```python
from build123d import *

# Parameters (mm, degrees)
BOSS_EXTRUDE1_DEPTH     = 22
SKETCH2_W               = 18.000000089
SKETCH2_H               = 20
BOSS_EXTRUDE2_DEPTH     = 7
SKETCH3_W               = 70
SKETCH3_H               = 50
BOSS_EXTRUDE3_DEPTH     = 4
SKETCH31_W              = 18.000000089
SKETCH31_H              = 3
BOSS_EXTRUDE7_DEPTH     = 34
CUT_EXTRUDE1_REACH      = 52
CUT_EXTRUDE_THIN1_REACH = 72
SKETCH7_W               = 25.000000089
SKETCH7_H               = 30
SKETCH8_W               = 18.000000089
SKETCH8_H               = 23
CUT_EXTRUDE2_DEPTH      = 27.000000055
CUT_EXTRUDE2_DEPTH_BACK = 45.000000145
SKETCH10_R              = 1
CUT_EXTRUDE3_DEPTH      = 10
SKETCH12_W              = 4
SKETCH12_H              = 5
CUT_EXTRUDE4_DEPTH      = 4
SKETCH13_W              = 18.000000089
SKETCH13_H              = 23
BOSS_EXTRUDE4_DEPTH     = 5
SKETCH14_R              = 1
CUT_EXTRUDE5_DEPTH      = 10
CUT_EXTRUDE6_REACH      = 40
CUT_EXTRUDE10_START     = -17
SKETCH29_W              = 13
SKETCH29_H              = 23
CUT_EXTRUDE10_DEPTH     = 17
SKETCH30_W              = 4
SKETCH30_H              = 1
CUT_EXTRUDE11_DEPTH     = 7
SKETCH21_R              = 5
CUT_EXTRUDE12_DEPTH     = 6
SKETCH32_R              = 4.999999958
BOSS_EXTRUDE8_DEPTH     = 2
CUT_EXTRUDE13_REACH     = 44.05
SKETCH33_R              = 1.5
SKETCH34_R              = 2.5
CUT_EXTRUDE14_DEPTH     = 1


with BuildPart() as part:
    # Sketch1 → Boss-Extrude1 (new body)
    with BuildSketch(Plane.XZ.offset(109.542579658)):
        Polygon((23.483775445, -24.37606884), (23.483775445, -44.37606884), (5.483775356, -44.37606884), (5.483775356, -24.37606884), (8.483775356, -24.37606884), (8.483775445, -41.37606884), (20.483775445, -41.37606884), (20.483775445, -24.37606884), align=None)
    extrude(amount=-BOSS_EXTRUDE1_DEPTH)

    # Sketch2 → Boss-Extrude2 (add)
    with BuildSketch(Plane.XZ.offset(109.542579658)):
        with Locations((14.483775401, -34.37606884)):
            Rectangle(SKETCH2_W, SKETCH2_H)
    extrude(amount=BOSS_EXTRUDE2_DEPTH)

    # Sketch3 → Boss-Extrude3 (add)
    with BuildSketch(Plane.XZ.offset(116.542579658)):
        with Locations((14.4837754, -26.325627156)):
            Rectangle(SKETCH3_W, SKETCH3_H)
    extrude(amount=BOSS_EXTRUDE3_DEPTH)

    # Sketch31 → Boss-Extrude7 (add)
    with BuildSketch(Plane(origin=(0, -116.542579658, 0), x_dir=(1, 0, 0), z_dir=(0, 1, 0))):
        with Locations((14.483775401, 45.87606884)):
            Rectangle(SKETCH31_W, SKETCH31_H)
    extrude(amount=BOSS_EXTRUDE7_DEPTH)

    # Sketch4 → Cut-Extrude1 (cut, up to next)
    with BuildSketch(Plane(origin=(0, 0, -51.325627156), x_dir=(-1, 0, 0), z_dir=(0, 0, -1)), mode=Mode.PRIVATE) as cut_extrude1_sk1:
        with BuildLine():
            Line((-49.4837754, -117.542579658), (-49.4837754, -120.542579658))
            Line((-49.4837754, -120.542579658), (-46.4837754, -120.542579658))
            ThreePointArc((-46.4837754, -120.542579658), (-48.605095744, -119.663900001), (-49.4837754, -117.542579658))
        make_face()
    cut_extrude1_tool1 = extrude(cut_extrude1_sk1.sketch, amount=-CUT_EXTRUDE1_REACH, mode=Mode.PRIVATE) & part.part
    add(cut_extrude1_tool1.solids().sort_by_distance((48.813672, -119.872476, -51.325627))[0], mode=Mode.SUBTRACT)
    # Sketch4 → Cut-Extrude1 (cut, up to next)
    with BuildSketch(Plane(origin=(0, 0, -51.325627156), x_dir=(-1, 0, 0), z_dir=(0, 0, -1)), mode=Mode.PRIVATE) as cut_extrude1_sk2:
        with BuildLine():
            Line((17.5162246, -120.542579658), (20.5162246, -120.542579658))
            Line((20.5162246, -120.542579658), (20.5162246, -117.542579658))
            ThreePointArc((20.5162246, -117.542579658), (19.637544943, -119.663900001), (17.5162246, -120.542579658))
        make_face()
    cut_extrude1_tool2 = extrude(cut_extrude1_sk2.sketch, amount=-CUT_EXTRUDE1_REACH, mode=Mode.PRIVATE) & part.part
    add(cut_extrude1_tool2.solids().sort_by_distance((-19.846121, -119.872476, -51.325627))[0], mode=Mode.SUBTRACT)

    # Sketch6 → Cut-Extrude-Thin1 (cut, up to next)
    with BuildSketch(Plane.ZY.offset(20.5162246), mode=Mode.PRIVATE) as cut_extrude_thin1_sk1:
        with BuildLine():
            ThreePointArc((-4.325627156, -120.542579658), (-2.204306812, -119.663900001), (-1.325627156, -117.542579658))
            Line((-1.325627156, -117.542579658), (8.674372844, -117.542579658))
            ThreePointArc((8.674372844, -117.542579658), (4.866761, -126.734967813), (-4.325627156, -130.542579658))
            Line((-4.325627156, -130.542579658), (-4.325627156, -120.542579658))
        make_face()
    cut_extrude_thin1_tool1 = extrude(cut_extrude_thin1_sk1.sketch, amount=-CUT_EXTRUDE_THIN1_REACH, mode=Mode.PRIVATE) & part.part
    add(cut_extrude_thin1_tool1.solids().sort_by_distance((-20.516225, -123.298683, 1.430477))[0], mode=Mode.SUBTRACT)
    # Sketch6 → Cut-Extrude-Thin1 (cut, up to next)
    with BuildSketch(Plane.ZY.offset(20.5162246), mode=Mode.PRIVATE) as cut_extrude_thin1_sk2:
        with BuildLine():
            ThreePointArc((-51.325627156, -117.542579658), (-50.446947499, -119.663900001), (-48.325627156, -120.542579658))
            Line((-48.325627156, -120.542579658), (-48.325627156, -130.542579658))
            ThreePointArc((-48.325627156, -130.542579658), (-57.518015311, -126.734967813), (-61.325627156, -117.542579658))
            Line((-61.325627156, -117.542579658), (-51.325627156, -117.542579658))
        make_face()
    cut_extrude_thin1_tool2 = extrude(cut_extrude_thin1_sk2.sketch, amount=-CUT_EXTRUDE_THIN1_REACH, mode=Mode.PRIVATE) & part.part
    add(cut_extrude_thin1_tool2.solids().sort_by_distance((-20.516225, -123.298683, -54.081731))[0], mode=Mode.SUBTRACT)

    # Sketch7 → Loft2 section 0
    with BuildSketch(Plane(origin=(0, -116.542579658, 0), x_dir=(1, 0, 0), z_dir=(0, 1, 0))):
        with Locations((14.483775401, 35.87606884)):
            Rectangle(SKETCH7_W, SKETCH7_H)
    # Sketch8 → Loft2 section 1
    with BuildSketch(Plane(origin=(0, -112.542579658, 0), x_dir=(1, 0, 0), z_dir=(0, 1, 0))):
        with Locations((14.483775401, 35.87606884)):
            Rectangle(SKETCH8_W, SKETCH8_H)
    loft()

    # Sketch9 → Cut-Extrude2 (cut, two sides)
    with BuildSketch(Plane.ZY.offset(-5.483775356)) as cut_extrude2_sk:
        Polygon((-24.37606884, -112.542579658), (-24.37606884, -116.542579658), (-20.87606884, -116.542579658), align=None)
    extrude(amount=CUT_EXTRUDE2_DEPTH, mode=Mode.SUBTRACT)
    extrude(cut_extrude2_sk.sketch, amount=-CUT_EXTRUDE2_DEPTH_BACK, mode=Mode.SUBTRACT)

    # Sketch10 → Cut-Extrude3 (cut)
    with BuildSketch(Plane.XY.offset(-24.37606884)):
        with Locations((14.483775445, -112.542579896)):
            Circle(SKETCH10_R)
    extrude(amount=-CUT_EXTRUDE3_DEPTH, mode=Mode.SUBTRACT)

    # Sketch12 → Cut-Extrude4 (cut)
    with BuildSketch(Plane.XY.offset(-34.37606884)):
        with Locations((14.483775445, -112.042579658)):
            Rectangle(SKETCH12_W, SKETCH12_H)
    extrude(amount=CUT_EXTRUDE4_DEPTH, mode=Mode.SUBTRACT)

    # Sketch13 → Boss-Extrude4 (add)
    with BuildSketch(Plane(origin=(0, -87.542579658, 0), x_dir=(1, 0, 0), z_dir=(0, 1, 0))):
        with Locations((14.483775401, 35.87606884)):
            Rectangle(SKETCH13_W, SKETCH13_H)
    extrude(amount=BOSS_EXTRUDE4_DEPTH)

    # Sketch14 → Cut-Extrude5 (cut)
    with BuildSketch(Plane.XY.offset(-24.37606884)):
        with Locations((14.483775445, -84.542579419)):
            Circle(SKETCH14_R)
    extrude(amount=-CUT_EXTRUDE5_DEPTH, mode=Mode.SUBTRACT)

    # Sketch16 → Cut-Extrude6 (cut, up to next)
    with BuildSketch(Plane(origin=(0, -82.542579658, 0), x_dir=(1, 0, 0), z_dir=(0, 1, 0)), mode=Mode.PRIVATE) as cut_extrude6_sk1:
        Polygon((14.4837754, 41.37606884), (8.4837754, 41.37606884), (8.4837754, 31.37606884), (20.4837754, 31.37606884), (20.4837754, 41.37606884), align=None)
    cut_extrude6_tool1 = extrude(cut_extrude6_sk1.sketch, amount=-CUT_EXTRUDE6_REACH, mode=Mode.PRIVATE) & part.part
    add(cut_extrude6_tool1.solids().sort_by_distance((14.483775, -82.54258, -36.376069))[0], mode=Mode.SUBTRACT)

    # Sketch29 → Cut-Extrude10 (cut)
    with BuildSketch(Plane.XY.offset(-24.37606884).offset(CUT_EXTRUDE10_START)):
        with Locations((14.483775445, -98.542579658)):
            Rectangle(SKETCH29_W, SKETCH29_H)
    extrude(amount=CUT_EXTRUDE10_DEPTH, mode=Mode.SUBTRACT)

    # Sketch30 → Cut-Extrude11 (cut)
    with BuildSketch(Plane.XY.offset(-24.37606884)):
        with Locations((14.483775445, -86.542579658)):
            Rectangle(SKETCH30_W, SKETCH30_H)
    extrude(amount=-CUT_EXTRUDE11_DEPTH, mode=Mode.SUBTRACT)

    # Sketch21 → Cut-Extrude12 (cut)
    with BuildSketch(Plane.XY.offset(-41.37606884)):
        with Locations((14.4837754, -93.542579583)):
            Circle(SKETCH21_R)
    extrude(amount=-CUT_EXTRUDE12_DEPTH, mode=Mode.SUBTRACT)

    # Sketch32 → Boss-Extrude8 (add)
    with BuildSketch(Plane.XY.offset(-41.37606884)):
        with Locations((14.483775445, -93.542579583)):
            Circle(SKETCH32_R)
    extrude(amount=-BOSS_EXTRUDE8_DEPTH)

    # Sketch33 → Cut-Extrude13 (cut, up to next)
    with BuildSketch(Plane(origin=(0, 0, -43.37606884), x_dir=(-1, 0, 0), z_dir=(0, 0, -1)), mode=Mode.PRIVATE) as cut_extrude13_sk1:
        with Locations((-14.4837754, -93.542579583)):
            Circle(SKETCH33_R)
    cut_extrude13_tool1 = extrude(cut_extrude13_sk1.sketch, amount=-CUT_EXTRUDE13_REACH, mode=Mode.PRIVATE) & part.part
    add(cut_extrude13_tool1.solids().sort_by_distance((14.483775, -93.54258, -43.376069))[0], mode=Mode.SUBTRACT)

    # Sketch34 → Cut-Extrude14 (cut)
    with BuildSketch(Plane.XY.offset(-41.37606884)):
        with Locations((14.4837754, -93.542579583)):
            Circle(SKETCH34_R)
    extrude(amount=-CUT_EXTRUDE14_DEPTH, mode=Mode.SUBTRACT)


solid = part.part
```
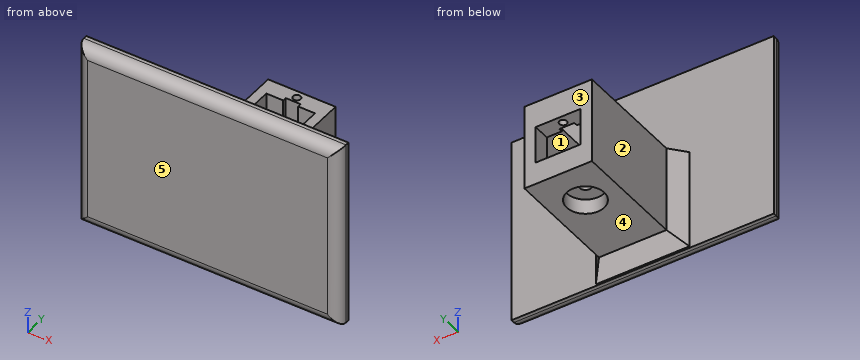
The listing builds one solid part. Answer for the finished solid, in the listing's coordinates (mm). Face numbers are marked on the shaded views. A direction names the side the tool comes from. Coordinates: 2 decimals unless noted, no trailing zeros. Loops run counter-clockwise (first coordinate to the right, second up) from the corner with the lowest first, then second, coordinate; pieces in that order, holes last. Notation, with made-up numbers: M 55.25,35 L 106.25,35 A17 ccw 106.25,55 Z; hole C -17,17 d3. An arc over 180 degrees is marked long. Answer as CSV lines item,"result". Start each with the question number.
(1) Find the intervals of material crossed by L1, parallel to X at y = -91, z = -31; L2, parallel to Y at x = -5, z = -37; L3, parallel to X at y = -111, z = -37, in increasing order. Write a range as [from, to].
(2) The part is cut by section C-C (x = 35.5). Give the vertices of the cut face in (y, z).
(3) The part is cut by section A-A (y = -101). Give the vertices of the cut face in (x, z).
(4) The part is cut by section B-B (z = -13.5). Give the vertices of the cut face in (x, y).
(5) The mould has two halves that part along X. Classify the marked faces 1, 2 and 3: pulls with the +X half, pulls with the -X half, needs draft (parallel to the pull), parting line crosses it, or undercut.
(6) Given pin 1 (6.5 mm diameter, centred on x = 13.5, z = -36.5, fed in from +Y); pin 2 (6.5 mm diameter, centred on x = 14.48, y = -93.54, fed in from -Z); pin 3 (5 mm diameter, centred on x = 22.5, z = -10.5, fed in from +Y); pin 4 (8 mm diameter, centred on y = -94.5, z = -19.5, fed in from -X), each flat-ended and moving along its own axis, determine where each tip first touches the part or whether it passes through.
(7) For the marked faces 4 and 5, determine the directions among +Z, -Z, +X, -X, +Y, -Y from which every point of the face is accessible in a straight line to the end or side of a thin tool.
(8) The part is cut by section D-D (z = -29). State how many separate pieces and enclosed holes the cut face has, and give its area (3 significant figures).
Determined:
1,L1,"[5.48, 7.98], [20.98, 23.48]"
1,L2,"[-120.54, -116.54]"
1,L3,"[5.48, 23.48]"
2,outline,"M -120.54,-48.33 A3 ccw -117.54,-51.33 L -116.54,-51.33 L -116.54,-1.33 L -117.54,-1.33 A3 ccw -120.54,-4.33 Z"
3,outline,"M 5.48,-47.38 L 23.48,-47.38 L 23.48,-24.38 L 20.98,-24.38 L 20.98,-41.38 L 7.98,-41.38 L 7.98,-24.38 L 5.48,-24.38 Z"
4,outline,"M -20.52,-117.54 A3 ccw -17.52,-120.54 L 46.48,-120.54 A3 ccw 49.48,-117.54 L 49.48,-116.54 L -20.52,-116.54 Z"
5,face 1,"undercut"
5,face 2,"pulls with the -X half"
5,face 3,"needs draft"
6,pin 1,"y = -110.04"
6,pin 2,"z = -43.38"
6,pin 3,"y = -116.54"
6,pin 4,"through"
7,face 4,"-Z, +X, -X, +Y"
7,face 5,"+Z, -Z, +X, -X, -Y"
8,separate pieces,"1"
8,enclosed holes,"3"
8,area,"593 mm2"
